Design review of the part built by this model. Coordinates are the model's own, in mm. A direction names the side the tool comes from. Give positions to 0.01 mm unless a question says otherwise; leave off trailing zeros. Loops run counter-clockwise (first coordinate to the right, second up) from the corner with the lowest first, then second, coordinate; pieces in that order, holes last. Notation, with made-up numbers: (-23, -10) -> (34, -10) arc R18 ccw to (34, 4) -> close; hole circle Ø9 at (46, -20.75). An arc over 180 degrees is marked (long way). Answer in a Markdown table with one row per item. Add a question column.
(1) For faces 1 (the cylindrical face through (13.317, -5.028, 1.517)), 2 (the flat face through (3, -2, 0)), 3 (the flat face through (4, 3, 1)), 4 (the flat face through (-10, 0, -8.1)), list the 3-axis set-ups (+Z, -Z, +X, -X, +Y, -Y) from which the entire face can be reached by the end or side of a thin tool; tool diameter is ignored.
(2) Draft analysis for pull direction X (two halves, no side actions). For faces 5 (the cylindrical face through (13.138, 2.507, 6.518)), 6 (the cylindrical face through (4.2, -2.5, -0.1)), 7 (the flat face through (15, 3, 0)), state which applies: +X half, -X half, draft (parallel to the pull), parting line (faces both ways), or undercut.
(3) For pin 1 (8 mm diameter, centred on y = 2.5, z = -14.5, fed in from +X); pin 2 (5 mm diameter, centred on x = 7.5, z = -2, fed in from -Y); pin 3 (1 mm diameter, centred on y = 2, z = 4.5, fed in from -X), all flat-tipped, find the tip position at first contact; note any pin that passes through.
(4) Consider section A-A on z = 0. Write out the cut boundary in (x, y).
(5) Consider section D-D on y = 1.25. Write out the cut boundary in (x, z), then the cut area to 3 significant figures.
(6) Consider section C-C on z = -14.5. Write out the cut boundary in (x, y).
(7) Consider section B-B on x = -9. Write out the cut boundary in (y, z), then the cut area to 3 significant figures.
(8) For line 1 (Y direction, x = 4.5, z = -6.25); line 2 (Z direction, x = 8.5, y = -4.4); line 3 (X direction, y = 3, z = -14.25), list the stretches that pass through material, from the lowest coordinate up.
from build123d import *

# Parameters (mm, degrees)
SKETCH1_W           = 18
SKETCH1_H           = 16
BOSS_EXTRUDE1_DEPTH = 7
SKETCH4_W           = 16
SKETCH4_H           = 10.1
CUT_EXTRUDE1_DEPTH  = 16.1
SKETCH5_R           = 5.05
BOSS_EXTRUDE2_DEPTH = 4
SKETCH7_W           = 18
SKETCH7_H           = 1.95
BOSS_EXTRUDE3_DEPTH = 10
SKETCH8_R           = 1.5
CUT_EXTRUDE2_DEPTH  = 1.95
BOSS_EXTRUDE4_DEPTH = 1
SKETCH10_R          = 1.55
CUT_EXTRUDE3_DEPTH  = 14
SKETCH13_W          = 18
SKETCH13_H          = 12.05
BOSS_EXTRUDE6_DEPTH = 2
BOSS_EXTRUDE7_DEPTH = 2
SKETCH15_W          = 16.1
SKETCH15_H          = 10.1
CUT_EXTRUDE4_DEPTH  = 0.1


with BuildPart() as part:
    # Sketch1 → Boss-Extrude1 (new body, symmetric)
    with BuildSketch(Plane(origin=(0, 0, 0), x_dir=(1, 0, 0), z_dir=(0, 1, 0))):
        with Locations((-9, 0)):
            Rectangle(SKETCH1_W, SKETCH1_H)
    extrude(amount=BOSS_EXTRUDE1_DEPTH, both=True)

    # Sketch4 → Cut-Extrude1 (cut)
    with BuildSketch(Plane.ZY.offset(18)):
        Rectangle(SKETCH4_W, SKETCH4_H)
    extrude(amount=-CUT_EXTRUDE1_DEPTH, mode=Mode.SUBTRACT)

    # Sketch5 → Boss-Extrude2 (add)
    with BuildSketch(Plane.XZ.offset(7)):
        with BuildLine():
            Line((0, 8), (8.5, 8.05))
            ThreePointArc((8.5, 8.05), (16.55, 0), (8.5, -8.05))
            Line((8.5, -8.05), (0, -8))
            Line((0, -8), (0, 8))
        make_face()
        with Locations((8.5, 0)):
            Circle(SKETCH5_R, mode=Mode.SUBTRACT)
    boss_extrude2 = extrude(amount=-BOSS_EXTRUDE2_DEPTH)

    # Mirror1: Boss-Extrude2 across plane
    add(boss_extrude2.mirror(Plane(origin=(0, 0, 0), x_dir=(0, 0, 1), z_dir=(0, -1, 0))))

    # Sketch7 → Boss-Extrude3 (add)
    with BuildSketch(Plane(origin=(0, 0, -8), x_dir=(-1, 0, 0), z_dir=(0, 0, -1))):
        with Locations((9, 6.025)):
            Rectangle(SKETCH7_W, SKETCH7_H)
    extrude(amount=BOSS_EXTRUDE3_DEPTH)

    # Sketch8 → Cut-Extrude2 (cut)
    with BuildSketch(Plane.XZ.offset(-7)):
        with Locations((-9, -14.5)):
            Circle(SKETCH8_R)
    extrude(amount=CUT_EXTRUDE2_DEPTH, mode=Mode.SUBTRACT)

    # Sketch9 → Boss-Extrude4 (add)
    with BuildSketch(Plane(origin=(0, -3, 0), x_dir=(1, 0, 0), z_dir=(0, 1, 0))):
        with BuildLine():
            Line((11.805676935, -2.75), (16.012489601, -2.75))
            ThreePointArc((16.012489601, -2.75), (13.082575695, -6.557438524), (8.5, -8))
            Line((8.5, -8), (0, -8))
            Line((0, -8), (0, 8))
            Line((0, 8), (8.5, 8))
            ThreePointArc((8.5, 8), (13.082575695, 6.557438524), (16.012489601, 2.75))
            Line((16.012489601, 2.75), (11.805676935, 2.75))
            ThreePointArc((11.805676935, 2.75), (4.2, 0), (11.805676935, -2.75))
        make_face()
    boss_extrude4 = extrude(amount=BOSS_EXTRUDE4_DEPTH)

    # Mirror2: Boss-Extrude4 across plane
    add(boss_extrude4.mirror(Plane(origin=(0, 0, 0), x_dir=(0, 0, 1), z_dir=(0, -1, 0))))

    # Sketch10 → Cut-Extrude3 (cut)
    with BuildSketch(Plane.XZ.offset(7)):
        with Locations((-10, 2)):
            Circle(SKETCH10_R)
    extrude(amount=-CUT_EXTRUDE3_DEPTH, mode=Mode.SUBTRACT)

    # Sketch13 → Boss-Extrude6 (add)
    with BuildSketch(Plane(origin=(0, 0, -8), x_dir=(-1, 0, 0), z_dir=(0, 0, -1))):
        with Locations((9, -0.975)):
            Rectangle(SKETCH13_W, SKETCH13_H)
    extrude(amount=BOSS_EXTRUDE6_DEPTH)

    # Sketch14 → Boss-Extrude7 (add)
    with BuildSketch(Plane(origin=(0, 0, 0), x_dir=(0, 0, -1), z_dir=(1, 0, 0))):
        Polygon((10, -7), (18, 5.05), (10, 5.05), align=None)
    boss_extrude7 = extrude(amount=-BOSS_EXTRUDE7_DEPTH)

    # Mirror3: Boss-Extrude7 across plane
    add(boss_extrude7.mirror(Plane(origin=(-9, 0, 0), x_dir=(0, 0, 1), z_dir=(1, 0, 0))))

    # Sketch15 → Cut-Extrude4 (cut)
    with BuildSketch(Plane.XY.offset(-8)):
        with Locations((-9.95, 0)):
            Rectangle(SKETCH15_W, SKETCH15_H)
    extrude(amount=-CUT_EXTRUDE4_DEPTH, mode=Mode.SUBTRACT)


solid = part.part
Values follow:
| question | item | result |
|---|---|---|
| 1 | face 1 | -Y |
| 1 | face 2 | +Z, -Z, +X |
| 1 | face 3 | +Y |
| 1 | face 4 | +Z, -X |
| 2 | face 5 | +X half |
| 2 | face 6 | undercut |
| 2 | face 7 | draft |
| 3 | pin 1 | x = 0 |
| 3 | pin 2 | y = -3 |
| 3 | pin 3 | x = -1.9 |
| 4 | outline | (-18, -7) -> (3.45, -7) -> (3.45, -3) -> (4.2, -3) -> (4.2, -2) -> (0, -2) -> (0, 2) -> (4.2, 2) -> (4.2, 3) -> (3.45, 3) -> (3.45, 7) -> (-18, 7) -> (-18, 5.05) -> (-1.9, 5.05) -> (-1.9, -5.05) -> (-18, -5.05) -> close; (13.55, -7) -> (16.55, -7) -> (16.55, -3) -> (13.55, -3) -> close; (13.55, 3) -> (16.55, 3) -> (16.55, 7) -> (13.55, 7) -> close |
| 5 | outline | (-18, -15.48) -> (-16, -15.48) -> (-16, -10) -> (-2, -10) -> (-2, -15.48) -> (0, -15.48) -> (0, 8) -> (-1.9, 8) -> (-1.9, -8.1) -> (-18, -8.1) -> close |
| 5 | area | 86.7 mm2 |
| 6 | outline | (-18, -0.22) -> (-16, -0.22) -> (-16, 5.05) -> (-10.5, 5.05) -> (-10.5, 7) -> (-18, 7) -> close; (-7.5, 5.05) -> (-2, 5.05) -> (-2, -0.22) -> (0, -0.22) -> (0, 7) -> (-7.5, 7) -> close |
| 7 | outline | (-7, -10) -> (5.05, -10) -> (5.05, -13) -> (7, -13) -> (7, 0.82) -> (5.05, 0.82) -> (5.05, -8.1) -> (-5.05, -8.1) -> (-5.05, 0.82) -> (-7, 0.82) -> close; (-7, 3.18) -> (-5.05, 3.18) -> (-5.05, 8) -> (-7, 8) -> close; (5.05, -18) -> (7, -18) -> (7, -16) -> (5.05, -16) -> close; (5.05, 3.18) -> (7, 3.18) -> (7, 8) -> (5.05, 8) -> close |
| 7 | area | 89.9 mm2 |
| 8 | line 1 | -7 to -2, 2 to 7 |
| 8 | line 2 | -8.05 to -5.05, 5.05 to 8.05 |
| 8 | line 3 | -18 to -16, -2 to 0 |
